Autodesk Inventor part; units mm, degrees
ref_plane "Work Plane1" through (0, 0, 28.575) normal (0, 0, 1) x (1, 0, 0)
ref_plane "YZ Plane" through (0, 0, 0) normal (1, 0, 0) x (0, 1, 0)
ref_plane "XZ Plane" through (0, 0, 0) normal (0, 1, 0) x (-1, 0, 0)
sketch "Sketch1" plane through (0, 0, 0) normal (0, 0, 1) x (1, 0, 0)
  line L0 (17.78, -10.2653) -> (0, -20.5306)
  line L1 (0, -20.5306) -> (-17.78, -10.2653)
  line L2 (-17.78, -10.2653) -> (-17.78, 10.2653)
  line L3 (-17.78, 10.2653) -> (0, 20.5306)
  line L4 (0, 20.5306) -> (17.78, 10.2653)
  line L5 (17.78, 10.2653) -> (17.78, -10.2653)
  line L6 (0, 0) -> (20.8337, 0) construction
  line L7 (57.15, -10.2653) -> (39.37, -20.5306)
  line L8 (39.37, -20.5306) -> (21.59, -10.2653)
  line L9 (21.59, -10.2653) -> (21.59, 10.2653)
  line L10 (21.59, 10.2653) -> (39.37, 20.5306)
  line L11 (39.37, 20.5306) -> (57.15, 10.2653)
  line L12 (57.15, 10.2653) -> (57.15, -10.2653)
  line L13 (39.37, 0) -> (60.2037, 0) construction
  line L14 (96.52, -10.2653) -> (78.74, -20.5306)
  line L15 (78.74, -20.5306) -> (60.96, -10.2653)
  line L16 (60.96, -10.2653) -> (60.96, 10.2653)
  line L17 (60.96, 10.2653) -> (78.74, 20.5306)
  line L18 (78.74, 20.5306) -> (96.52, 10.2653)
  line L19 (96.52, 10.2653) -> (96.52, -10.2653)
  line L20 (78.74, 0) -> (99.5737, 0) construction
  line L21 (135.89, -10.2653) -> (118.11, -20.5306)
  line L22 (118.11, -20.5306) -> (100.33, -10.2653)
  line L23 (100.33, -10.2653) -> (100.33, 10.2653)
  line L24 (100.33, 10.2653) -> (118.11, 20.5306)
  line L25 (118.11, 20.5306) -> (135.89, 10.2653)
  line L26 (135.89, 10.2653) -> (135.89, -10.2653)
  line L27 (118.11, 0) -> (138.9437, 0) construction
  line L28 (175.26, -10.2653) -> (157.48, -20.5306)
  line L29 (157.48, -20.5306) -> (139.7, -10.2653)
  line L30 (139.7, -10.2653) -> (139.7, 10.2653)
  line L31 (139.7, 10.2653) -> (157.48, 20.5306)
  line L32 (157.48, 20.5306) -> (175.26, 10.2653)
  line L33 (175.26, 10.2653) -> (175.26, -10.2653)
  line L34 (157.48, 0) -> (178.3137, 0) construction
  line L35 (-17.78, 0) -> (-21.59, 0) construction
  line L36 (0, -20.5306) -> (0, -24.3406) construction
  line L37 (0, -24.3406) -> (-21.59, -24.3406) construction
  line L38 (-21.59, -24.3406) -> (-21.59, 0) construction
  line L39 (157.48, -20.5306) -> (157.48, -24.3406) construction
  line L40 (175.26, 0) -> (179.07, 0) construction
  line L41 (179.07, 0) -> (179.07, -24.3406) construction
  line L42 (179.07, -24.3406) -> (157.48, -24.3406) construction
  line L43 (-17.78, 0) -> (-21.59, 0)
  line L44 (-21.59, -24.3406) -> (-21.59, 0)
  line L45 (-21.59, -24.3406) -> (179.07, -24.3406)
  line L46 (179.07, -24.3406) -> (179.07, 0)
  line L47 (179.07, 0) -> (175.26, 0)
  line L48 (17.78, 0) -> (21.59, 0)
  line L49 (57.15, 0) -> (60.96, 0)
  line L50 (96.52, 0) -> (100.33, 0)
  line L51 (135.89, 0) -> (139.7, 0)
  dimension "d0" = 35.56
  dimension "d3" = 39.37
  dimension "d8" = 3.81
  dimension "d9" = 3.81
  dimension "d10" = 3.81
  dimension "d11" = 3.81
extrude "Extrusion1" add sketch "Sketch1" along normal blind 57.15 contours L5 L48 L9 L8 L7 L12 L49 L16 L15 L14 L19 L50 L23 L22 L21 L26 L51 L30 L29 L28 L33 L47 L46 L45 L44 L43 L2 L1 L0
sketch "Sketch2" plane through (0, 0, 57.15) normal (0, 0, 1) x (1, 0, 0)
  line L0 (-17.78, -10.2653) -> (-17.78, 0) construction
  line L1 (-17.78, 0) -> (-21.59, 0) construction
  line L2 (-21.59, 0) -> (-21.59, -24.3406) construction
  line L3 (-21.59, -24.3406) -> (179.07, -24.3406) construction
  line L4 (179.07, -24.3406) -> (179.07, 0) construction
  line L5 (179.07, 0) -> (175.26, 0) construction
  line L6 (175.26, 0) -> (175.26, -10.2653) construction
  line L7 (175.26, -10.2653) -> (157.48, -20.5306) construction
  line L8 (157.48, -20.5306) -> (139.7, -10.2653) construction
  line L9 (139.7, -10.2653) -> (139.7, 0) construction
  line L10 (139.7, 0) -> (135.89, 0) construction
  line L11 (135.89, 0) -> (135.89, -10.2653) construction
  line L12 (135.89, -10.2653) -> (118.11, -20.5306) construction
  line L13 (118.11, -20.5306) -> (100.33, -10.2653) construction
  line L14 (100.33, -10.2653) -> (100.33, 0) construction
  line L15 (100.33, 0) -> (96.52, 0) construction
  line L16 (96.52, 0) -> (96.52, -10.2653) construction
  line L17 (96.52, -10.2653) -> (78.74, -20.5306) construction
  line L18 (78.74, -20.5306) -> (60.96, -10.2653) construction
  line L19 (60.96, -10.2653) -> (60.96, 0) construction
  line L20 (60.96, 0) -> (57.15, 0) construction
  line L21 (57.15, 0) -> (57.15, -10.2653) construction
  line L22 (57.15, -10.2653) -> (39.37, -20.5306) construction
  line L23 (39.37, -20.5306) -> (21.59, -10.2653) construction
  line L24 (21.59, -10.2653) -> (21.59, 0) construction
  line L25 (21.59, 0) -> (17.78, 0) construction
  line L26 (17.78, 0) -> (17.78, -10.2653) construction
  line L27 (17.78, -10.2653) -> (0, -20.5306) construction
  line L28 (0, -20.5306) -> (-17.78, -10.2653) construction
  line L29 (-21.59, -24.3406) -> (179.07, -24.3406)
  line L30 (179.07, -24.3406) -> (179.07, 0)
  line L31 (179.07, 0) -> (-21.59, 0)
  line L32 (-21.59, 0) -> (-21.59, -24.3406)
  point P0 (0, 0)
ref_plane "Work Plane1" through (0, 0, 28.575) normal (0, 0, 1) x (1, 0, 0)
extrude "Extrusion2" add sketch "Sketch2" along normal blind 3.81
mirror "Mirror1" about plane through (0, 0, 28.575) normal (0, 0, 1) of "Extrusion2"
properties part number "Bottom"
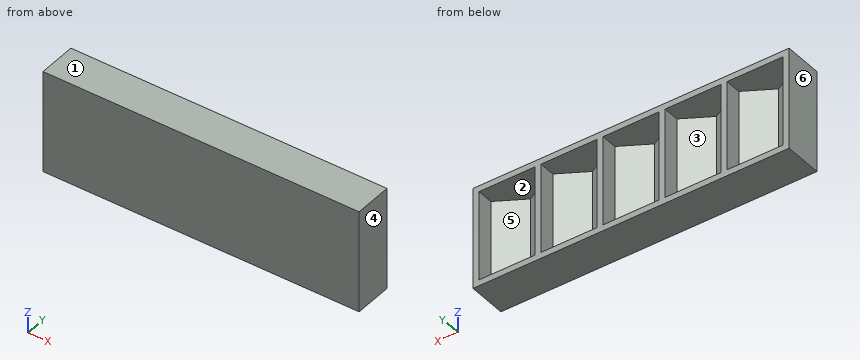
Can you work these out from the model? Positions are in its coordinate system, mm. Face numbers are marked on the shaded views. A direction names the side the tool comes from. Round coordinates to 2 decimals unless told otherwise and drop trailing zeros. Loops run counter-clockwise (first coordinate to the right, second up) from the corner with the lowest first, then second, coordinate; pieces in that order, holes last.
Item 1: If we mould it in two halves opening along X, with no side actions, what happens to the marked faces 1, 2, 3 and 4? For each: +X half, -X half, draft (parallel to the pull), parting line (faces both ways), or undercut.
Item 2: Suppose I cut it at A-A, the plane y = -6. Write out the boundary of the cut face in (x, z).
Item 3: Which directions (+Z, -Z, +X, -X, +Y, -Y) give clear straight access to the entire face, cutting with the end or side of a thin tool? Please do the marked faces 5 and 6.
Item 4: Suppose I cut it at C-C, the plane x = 162. Write out the boundary of the cut face in (y, z).
Item 5: Please list where these lines run through material, in increasing order: L1, parallel to X at y = -3.5, z = 13; L2, parallel to X at y = -12, z = 33; L3, parallel to Z at x = -3.5, y = -10.5.
Item 6: Will this pin go through, and if not, where does the flat tip stop? pin 1 Ø8 at (x, z) = (36.5, 51) entering from +Y.
Item 7: Suppose I cut it at D-D, the plane y = -18.5. Write out the boundary of the cut face in (x, z).
Reported:
1. face 1: draft
1. face 2: undercut
1. face 3: undercut
1. face 4: +X half
2. outline: (-21.59, -3.81) - (179.07, -3.81) - (179.07, 60.96) - (-21.59, 60.96) - close; hole (-17.78, 0) - (17.78, 0) - (17.78, 57.15) - (-17.78, 57.15) - close; hole (21.59, 0) - (57.15, 0) - (57.15, 57.15) - (21.59, 57.15) - close; hole (60.96, 0) - (96.52, 0) - (96.52, 57.15) - (60.96, 57.15) - close; hole (100.33, 0) - (135.89, 0) - (135.89, 57.15) - (100.33, 57.15) - close; hole (139.7, 0) - (175.26, 0) - (175.26, 57.15) - (139.7, 57.15) - close
3. face 5: +Y
3. face 6: +Z, -Z, -X, +Y, -Y
4. outline: (-24.34, -3.81) - (0, -3.81) - (0, 0) - (-17.92, 0) - (-17.92, 57.15) - (0, 57.15) - (0, 60.96) - (-24.34, 60.96) - close
5. L1: x = -21.59 to -17.78, 17.78 to 21.59, 57.15 to 60.96, 96.52 to 100.33, 135.89 to 139.7, 175.26 to 179.07
5. L2: x = -21.59 to -14.78, 14.78 to 24.59, 54.15 to 63.96, 93.52 to 103.33, 132.89 to 142.7, 172.26 to 179.07
5. L3: z = -3.81 to 0, 57.15 to 60.96
6. pin 1: stops at y = -16.56
7. outline: (-21.59, -3.81) - (179.07, -3.81) - (179.07, 60.96) - (-21.59, 60.96) - close; hole (-3.52, 0) - (3.52, 0) - (3.52, 57.15) - (-3.52, 57.15) - close; hole (35.85, 0) - (42.89, 0) - (42.89, 57.15) - (35.85, 57.15) - close; hole (75.22, 0) - (82.26, 0) - (82.26, 57.15) - (75.22, 57.15) - close; hole (114.59, 0) - (121.63, 0) - (121.63, 57.15) - (114.59, 57.15) - close; hole (153.96, 0) - (161, 0) - (161, 57.15) - (153.96, 57.15) - close
